from build123d import *

# Parameters (mm, degrees)
BOSS_EXTRUDE1_DEPTH = 450
SHELL1_T            = -0.35


with BuildPart() as part:
    # Sketch1 → Boss-Extrude1 (new body)
    with BuildSketch(Plane(origin=(0, 0, 0), x_dir=(1, 0, 0), z_dir=(0, 1, 0))):
        with BuildLine():
            Line((-8, -13.856406461), (-175.0875, -303.26044577))
            ThreePointArc((-175.0875, -303.26044577), (0, -350.175), (175.0875, -303.26044577))
            Line((175.0875, -303.26044577), (8, -13.856406461))
            ThreePointArc((8, -13.856406461), (0, -16), (-8, -13.856406461))
        make_face()
    extrude(amount=BOSS_EXTRUDE1_DEPTH)

    # Shell1
    shell1_openings = [part.faces().sort_by_distance(p)[0] for p in [
        (0, 450, 170.822963058),
    ]]
    offset(amount=SHELL1_T, openings=shell1_openings, kind=Kind.INTERSECTION)


solid = part.part
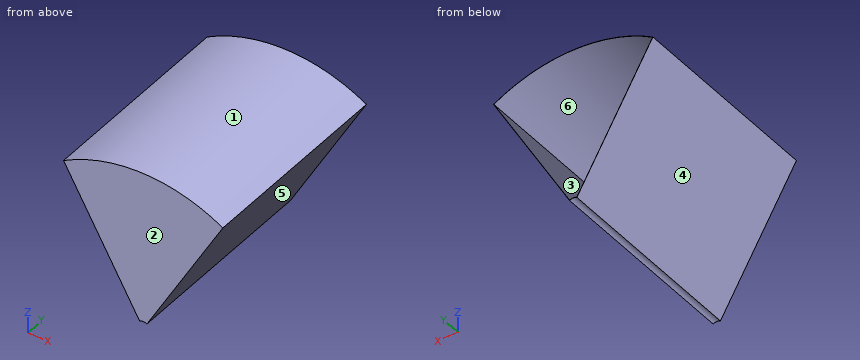
For this review, take the finished solid that the model builds, in its own axes (mm). Face numbers are marked on the shaded views. A direction names the side the tool comes from. Give positions to 0.01 mm unless a question says otherwise; leave off trailing zeros. Loops run counter-clockwise (first coordinate to the right, second up) from the corner with the lowest first, then second, coordinate; pieces in that order, holes last.
Item 1: Tool access review of the marked faces 5 and 6: name each direction out of +Z, -Z, +X, -X, +Y, -Y from which nothing blocks a thin tool from reaching the whole face with its end or side.
Item 2: For line 1 along Z through (x, y) = (-153, 138); line 2 along Z through (x, y) = (32.5, 150); line 3 along Y through (x, z) = (-93, 320.5), list the stretches that pass through material, from the lowest coordinate up.
Item 3: Take a section at C-C, the plane z = 66.5. State the section outline as (x, y) points, and give its area (3 significant figures).
Item 4: Insertion check: pin 1 (1 mm diameter, centred on y = 224.5, z = 128, fed in from -X); pin 2 (4 mm diameter, centred on y = 141.5, z = 179.5, fed in from -X); pin 3 (6 mm diameter, centred on x = 121.5, y = 181, fed in from +Z). Each pin has a flat end and moves straight along its axis. Give the tip position at first contact, or say it passes through.
Item 5: Draft analysis for pull direction Z (two halves, no side actions). For the marked faces 1, 2, 3 and 4, state which applies: +Z half, -Z half, draft (parallel to the pull), parting line (faces both ways), or undercut.
Item 6: Take a section at B-B, the plane x = -32. State the section outline as (y, z) points.
Calculated:
1. face 5: -Z, +X, +Y, -Y
1. face 6: +Y
2. line 1: z = 265 to 265.7, 314.59 to 314.98
2. line 2: z = 56.29 to 56.99, 348.31 to 348.66
2. line 3: y = 0 to 0.35
3. outline: (-38.39, 0) - (38.39, 0) - (38.39, 450) - (37.99, 450) - (37.99, 0.35) - (-37.99, 0.35) - (-37.99, 450) - (-38.39, 450) - close
3. area: 390 mm2
4. pin 1: stops at x = -74.19
4. pin 2: stops at x = -104.79
4. pin 3: stops at z = 329.52
5. face 1: +Z half
5. face 2: draft
5. face 3: undercut
5. face 4: -Z half
6. outline: (0, 55.43) - (450, 55.43) - (450, 56.13) - (0.35, 56.13) - (0.35, 348.36) - (450, 348.36) - (450, 348.71) - (0, 348.71) - close
